from build123d import *

# Parameters (mm, degrees)
SKETCH_1_R          = 1.531489915
EXTRUDE_1_DEPTH     = 1.68
SKETCH_1_R_2        = 1.063949022
EXTRUDE_1_2_DEPTH   = 1.68
SKETCH_1_R_3        = 2.489250022
EXTRUDE_1_3_DEPTH   = 1.68
SKETCH_1_W          = 72.86
SKETCH_1_H          = 61.86
SKETCH_1_R_4        = 1.55
EXTRUDE_1_4_DEPTH   = 1.68
SKETCH_2_R          = 3
SKETCH_2_R_2        = 1.55
EXTRUDE_3_DEPTH     = 2
SKETCH_3_W          = 72.86
SKETCH_3_H          = 61.86
SKETCH_3_W_2        = 69.50125591
SKETCH_3_H_2        = 58.5
EXTRUDE_4_DEPTH     = 15.85
SKETCH_4_W          = 17
SKETCH_4_H          = 15
CUT_EXTRUDE_1_DEPTH = 3.68
SKETCH_6_W          = 7.25
SKETCH_6_H          = 16
SKETCH_6_W_2        = 2.5
SKETCH_6_H_2        = 18
CUT_EXTRUDE_3_DEPTH = 7.8
SKETCH_7_W          = 10
SKETCH_7_H          = 4
SKETCH_7_W_2        = 17
SKETCH_7_H_2        = 8
SKETCH_7_W_3        = 8
SKETCH_7_H_3        = 13.300256909
CUT_EXTRUDE_5_DEPTH = 2
SKETCH_8_R          = 1.556852558
SKETCH_8_W          = 2.041099746
SKETCH_8_H          = 24.945353107
CUT_EXTRUDE_6_DEPTH = 2
FILLET_1_R          = 1.68
FILLET_2_R          = 2
FILLET_3_R          = 1.68
FILLET_4_R          = 2
FILLET_5_R          = 3
FILLET_6_R          = 1
FILLET_7_R          = 1
SKETCH_9_R          = 4
CUT_EXTRUDE_7_DEPTH = 0.8
SKETCH_10_W         = 44.758598589
SKETCH_10_H         = 6.5
SKETCH_10_W_2       = 44.448850503
CUT_EXTRUDE_8_DEPTH = 0.8
SKETCH_11_R         = 1.55
EXTRUDE_6_DEPTH     = 10.65
CUT_EXTRUDE_9_DEPTH = 62.6
FILLET_8_R          = 4
FILLET_9_R          = 1


with BuildPart() as part:
    # 草图1 → 凸台-拉伸1 (new body)
    with BuildSketch(Plane.XY):
        with Locations((1.504266973, 51.672660554)):
            Circle(SKETCH_1_R)
    extrude(amount=EXTRUDE_1_DEPTH)


with BuildPart() as body_2:
    # 草图1 → Extrude 1 2 (new body)
    with BuildSketch(Plane.XY):
        with Locations((-18.258772408, 61.840992468)):
            Circle(SKETCH_1_R_2)
    extrude(amount=EXTRUDE_1_2_DEPTH)


with BuildPart() as body_3:
    # 草图1 → Extrude 1 3 (new body)
    with BuildSketch(Plane.XY):
        with Locations((-18.258772408, -10.975845657)):
            Circle(SKETCH_1_R_3)
    extrude(amount=EXTRUDE_1_3_DEPTH)


with BuildPart() as body_4:
    # 草图1 → Extrude 1 4 (new body)
    with BuildSketch(Plane.XY):
        with Locations((-46.758772408, 26.672660554)):
            Rectangle(SKETCH_1_W, SKETCH_1_H)
        with Locations((-76.258772408, 51.672660554)):
            Circle(SKETCH_1_R_4, mode=Mode.SUBTRACT)
        with Locations((-18.258772408, 51.672660554)):
            Circle(SKETCH_1_R_4, mode=Mode.SUBTRACT)
        with Locations((-76.258772408, 2.672660554)):
            Circle(SKETCH_1_R_4, mode=Mode.SUBTRACT)
        with Locations((-18.258772408, 2.672660554)):
            Circle(SKETCH_1_R_4, mode=Mode.SUBTRACT)
    extrude(amount=EXTRUDE_1_4_DEPTH)

    # 草图2 → 凸台-拉伸3 (add)
    # profile 1 of 4: a face of its own
    with BuildSketch(Plane.XY.offset(1.68)):
        with Locations((-76.258772408, 2.672660554)):
            Circle(SKETCH_2_R)
        with Locations((-76.258772408, 2.672660554)):
            Circle(SKETCH_2_R_2, mode=Mode.SUBTRACT)
    # profile 2 of 4: a face of its own
    with BuildSketch(Plane.XY.offset(1.68)):
        with Locations((-18.258772408, 2.672660554)):
            Circle(SKETCH_2_R)
        with Locations((-18.258772408, 2.672660554)):
            Circle(SKETCH_2_R_2, mode=Mode.SUBTRACT)
    # profile 3 of 4: a face of its own
    with BuildSketch(Plane.XY.offset(1.68)):
        with Locations((-76.258772408, 51.672660554)):
            Circle(SKETCH_2_R)
        with Locations((-76.258772408, 51.672660554)):
            Circle(SKETCH_2_R_2, mode=Mode.SUBTRACT)
    # profile 4 of 4: a face of its own
    with BuildSketch(Plane.XY.offset(1.68)):
        with Locations((-18.258772408, 51.672660554)):
            Circle(SKETCH_2_R)
        with Locations((-18.258772408, 51.672660554)):
            Circle(SKETCH_2_R_2, mode=Mode.SUBTRACT)
    extrude(amount=EXTRUDE_3_DEPTH)

    # 草图3 → 凸台-拉伸4 (add)
    with BuildSketch(Plane.XY.offset(1.68)):
        with Locations((-46.758772408, 26.672660554)):
            Rectangle(SKETCH_3_W, SKETCH_3_H)
        with Locations((-46.758144453, 26.672660554)):
            Rectangle(SKETCH_3_W_2, SKETCH_3_H_2, mode=Mode.SUBTRACT)
    extrude(amount=EXTRUDE_4_DEPTH)

    # 草图4 → 切除-拉伸1 (cut)
    with BuildSketch(Plane(origin=(0, 0, 0), x_dir=(-1, 0, 0), z_dir=(0, 0, -1))):
        with Locations((74.688772408, 28.322197805)):
            Rectangle(SKETCH_4_W, SKETCH_4_H)
    extrude(amount=-CUT_EXTRUDE_1_DEPTH, mode=Mode.SUBTRACT)

    # 草图6 → 切除-拉伸3 (cut)
    with BuildSketch(Plane(origin=(-10.328772408, 0, 0), x_dir=(0, 0, -1), z_dir=(1, 0, 0))):
        with Locations((-8.625, 30.672660554)):
            Rectangle(SKETCH_6_W, SKETCH_6_H)
        with Locations((-14.975303343, 19.628822862)):
            Rectangle(SKETCH_6_W_2, SKETCH_6_H_2)
    extrude(amount=-CUT_EXTRUDE_3_DEPTH, mode=Mode.SUBTRACT)

    # 草图7 → 切除-拉伸5 (cut)
    with BuildSketch(Plane.XZ.offset(4.257339446)):
        with Locations((-69.258772408, 6.68)):
            Rectangle(SKETCH_7_W, SKETCH_7_H)
        with Locations((-47.758772408, 8.68)):
            Rectangle(SKETCH_7_W_2, SKETCH_7_H_2)
        with Locations((-26.258772408, 11.330128455)):
            Rectangle(SKETCH_7_W_3, SKETCH_7_H_3)
    extrude(amount=-CUT_EXTRUDE_5_DEPTH, mode=Mode.SUBTRACT)

    # 草图8 → 切除-拉伸6 (cut)
    with BuildSketch(Plane.ZY.offset(83.188772408)):
        with Locations((7.843859074, 9.687980695)):
            Circle(SKETCH_8_R)
        with Locations((7.730007332, 28.982792683)):
            Rectangle(SKETCH_8_W, SKETCH_8_H)
    extrude(amount=-CUT_EXTRUDE_6_DEPTH, mode=Mode.SUBTRACT)

    # 圆角1
    fillet_1_edges = [body_4.edges().sort_by_distance(p)[0] for p in [
        (-12.007516498, 55.922660554, 9.605),
        (-81.508772408, 55.922660554, 9.605),
        (-81.508772408, -2.577339446, 9.605),
        (-12.007516498, -2.577339446, 9.605),
        (-10.328772408, -4.257339446, 8.765),
        (-83.188772408, -4.257339446, 8.765),
        (-83.188772408, 57.602660554, 8.765),
        (-10.328772408, 57.602660554, 8.765),
    ]]
    fillet(fillet_1_edges, radius=FILLET_1_R)

    # 圆角2
    fillet_2_edges = [body_4.edges().sort_by_distance(p)[0] for p in [
        (-66.188772408, 20.822197805, 0.84),
        (-66.188772408, 35.822197805, 0.84),
    ]]
    fillet(fillet_2_edges, radius=FILLET_2_R)

    # 圆角3
    fillet_3_edges = [body_4.edges().sort_by_distance(p)[0] for p in [
        (-74.258772408, -3.417339446, 4.68),
        (-64.258772408, -3.417339446, 4.68),
    ]]
    fillet(fillet_3_edges, radius=FILLET_3_R)

    # 圆角4
    fillet_4_edges = [body_4.edges().sort_by_distance(p)[0] for p in [
        (-56.258772408, -3.417339446, 4.68),
        (-39.258772408, -3.417339446, 4.68),
    ]]
    fillet(fillet_4_edges, radius=FILLET_4_R)

    # 圆角5
    fillet_5_edges = [body_4.edges().sort_by_distance(p)[0] for p in [
        (-30.258772408, -3.417339446, 4.68),
        (-22.258772408, -3.417339446, 4.68),
    ]]
    fillet(fillet_5_edges, radius=FILLET_5_R)

    # 圆角6
    fillet_6_edges = [body_4.edges().sort_by_distance(p)[0] for p in [
        (-11.168144453, 10.628822862, 16.225303343),
        (-11.168144453, 28.628822862, 16.225303343),
        (-11.168144453, 28.628822862, 13.725303343),
        (-11.168144453, 10.628822862, 13.725303343),
    ]]
    fillet(fillet_6_edges, radius=FILLET_6_R)

    # 圆角7
    fillet_7_edges = [body_4.edges().sort_by_distance(p)[0] for p in [
        (-11.168144453, 38.672660554, 5),
        (-11.168144453, 22.672660554, 5),
        (-11.168144453, 22.672660554, 12.25),
        (-11.168144453, 38.672660554, 12.25),
        (-82.348772408, 16.510116129, 6.709457459),
        (-82.348772408, 41.455469236, 6.709457459),
        (-82.348772408, 41.455469236, 8.750557205),
        (-82.348772408, 16.510116129, 8.750557205),
        (-82.348772408, 20.822197805, 3.68),
        (-82.348772408, 35.822197805, 3.68),
    ]]
    fillet(fillet_7_edges, radius=FILLET_7_R)

    # 草图9 → 切除-拉伸7 (cut)
    with BuildSketch(Plane(origin=(0, 0, 0), x_dir=(-1, 0, 0), z_dir=(0, 0, -1))):
        with Locations((18.258772408, 51.672660554)):
            Circle(SKETCH_9_R)
        with Locations((76.258772408, 51.672660554)):
            Circle(SKETCH_9_R)
        with Locations((18.258772408, 2.672660554)):
            Circle(SKETCH_9_R)
        with Locations((76.258772408, 2.672660554)):
            Circle(SKETCH_9_R)
    extrude(amount=-CUT_EXTRUDE_7_DEPTH, mode=Mode.SUBTRACT)

    # 草图10 → 切除-拉伸8 (cut)
    with BuildSketch(Plane(origin=(0, 0, 0), x_dir=(-1, 0, 0), z_dir=(0, 0, -1))):
        with Locations((41.37196271, 38.672660554)):
            Rectangle(SKETCH_10_W, SKETCH_10_H)
        with Locations((41.37196271, 14.672660554)):
            Rectangle(SKETCH_10_W_2, SKETCH_10_H)
    extrude(amount=-CUT_EXTRUDE_8_DEPTH, mode=Mode.SUBTRACT)

    # 草图11 → 凸台-拉伸6 (add)
    # profile 1 of 2: a face of its own
    with BuildSketch(Plane.XY.offset(3.68)):
        Polygon((-79.828772408, 55.922660554), (-81.508772408, 54.242660554), (-81.508772408, 48.531036753), (-72.875228226, 48.531036753), (-72.875228226, 55.922660554), align=None)
        with Locations(Location((-76.258772408, 51.672660554, 0), (0, 0, 180))):
            Circle(SKETCH_11_R, mode=Mode.SUBTRACT)
    # profile 2 of 2: a face of its own
    with BuildSketch(Plane.XY.offset(3.68)):
        Polygon((-93.925658587, 53.936639744), (-95.605658587, 52.256639744), (-95.605658587, 46.545015943), (-86.972114405, 46.545015943), (-86.972114405, 53.936639744), align=None)
        with Locations(Location((-90.355658587, 49.686639744, 0), (0, 0, 180))):
            Circle(SKETCH_11_R, mode=Mode.SUBTRACT)
    extrude(amount=EXTRUDE_6_DEPTH)


with BuildPart() as extrude_6_piece_1:
    # of the separate pieces the step leaves, piece 1, a body of its own (extrude_6_pieces)
    add(body_4.part.solids().sort_by_distance((-10.328772408, 38.672660554, 6))[0])


with BuildPart() as extrude_6_piece_2:
    # of the separate pieces the step leaves, piece 2, a body of its own (extrude_6_pieces)
    add(body_4.part.solids().sort_by_distance((-93.925658587, 53.936639744, 3.68))[0])

    # 圆角8
    # the kernel refuses this fillet: 4 mm, written as the material it takes off along each edge
    with BuildSketch(Plane(origin=(-93.925658587, 53.936639744, -0.462135624), x_dir=(-0.7071067811865455, -0.7071067811865497, 0), z_dir=(0, 0, 1))) as fillet_8_piece_1:
        with BuildLine():
            CenterArc((FILLET_8_R * 0.414213562373, FILLET_8_R), FILLET_8_R, 225, 45)
            Line((-FILLET_8_R * 0.292893218813, FILLET_8_R * 0.292893218813), (0, 0))
            Line((0, 0), (FILLET_8_R * 0.414213562373, 0))
        make_face()
    extrude(amount=18.934271247, mode=Mode.SUBTRACT)
    with BuildSketch(Plane(origin=(-95.605658587, 52.256639744, -0.462135624), x_dir=(0.7071067811865411, 0.707106781186554, 0), z_dir=(0, 0, 1))) as fillet_8_piece_2:
        with BuildLine():
            CenterArc((FILLET_8_R * 0.414213562373, -FILLET_8_R), FILLET_8_R, 90, 45)
            Line((-FILLET_8_R * 0.292893218813, -FILLET_8_R * 0.292893218813), (0, 0))
            Line((0, 0), (FILLET_8_R * 0.414213562373, 0))
        make_face()
    extrude(amount=18.934271247, mode=Mode.SUBTRACT)

    # 圆角9
    fillet_9_edges = [extrude_6_piece_2.edges().sort_by_distance(p)[0] for p in [
        (-86.972114405, 53.936639744, 9.005),
        (-86.972114405, 46.545015943, 9.005),
        (-95.605658587, 46.545015943, 9.005),
    ]]
    fillet(fillet_9_edges, radius=FILLET_9_R)


with BuildPart() as cut_extrude_9_tool:
    # 草图13 → 切除-拉伸9 (new body)
    with BuildSketch(Plane.XY.offset(17.53)):
        Polygon((-85.534397359, 61.466506159), (-87.240895033, -11.116528255), (-1.802244806, -17.146153371), (14.580132867, 61.466506159), (-40.278079036, 71.546219088), align=None)
    extrude(amount=-CUT_EXTRUDE_9_DEPTH)


with BuildPart() as part_1:
    add(part.part)

    # 切除-拉伸9: cut by cut_extrude_9_tool
    add(cut_extrude_9_tool.part, mode=Mode.SUBTRACT)


with BuildPart() as body_2_1:
    add(body_2.part)

    # 切除-拉伸9: cut by cut_extrude_9_tool
    add(cut_extrude_9_tool.part, mode=Mode.SUBTRACT)


with BuildPart() as body_3_1:
    add(body_3.part)

    # 切除-拉伸9: cut by cut_extrude_9_tool
    add(cut_extrude_9_tool.part, mode=Mode.SUBTRACT)


with BuildPart() as extrude_6_piece_1_1:
    add(extrude_6_piece_1.part)

    # 切除-拉伸9: cut by cut_extrude_9_tool
    add(cut_extrude_9_tool.part, mode=Mode.SUBTRACT)


solid = extrude_6_piece_2.part
Could you check a few things on this model? Use its own coordinates, in mm. Give positions to 0.01 mm unless a question says otherwise; leave off trailing zeros. Order: outer loops, then holes, each group sorted by start corner. A loop starts at its lowest first (then second) coordinate and runs counter-clockwise, first axis right, second up.
1. Thinking about a two-plate mould opening in X: for faces 1 (the cylindrical face through (-91.834, 49.221, 8.93)), 2 (the flat face through (-91, 46.545, 9)), 3 (the cylindrical face through (-87.257, 46.846, 9.08)), which applies, +X half, -X half, draft (parallel to the pull), parting line (faces both ways), or undercut?
Answers below:
face 1: undercut
face 2: draft
face 3: +X half
2. Suppose I cut it at A-A (x = -89.25). Write out the boundary of the cut face in (y, z), plus the area to 3 significant figures.
Answers below:
outline: (46.55, 3.68) - (48.6, 3.68) - (48.6, 14.33) - (46.55, 14.33) - close; (50.77, 3.68) - (53.94, 3.68) - (53.94, 14.33) - (50.77, 14.33) - close
area: 55.6 mm2
3. Suppose I cut it at B-B (y = 49.25). Write out the boundary of the cut face in (x, z).
Answers below:
outline: (-95.61, 3.68) - (-91.84, 3.68) - (-91.84, 14.33) - (-95.61, 14.33) - close; (-88.87, 3.68) - (-86.97, 3.68) - (-86.97, 14.33) - (-88.87, 14.33) - close
4. Suppose I cut it at D-D (y = 52.75). Write out the boundary of the cut face in (x, z).
Answers below:
outline: (-94.98, 3.68) - (-86.97, 3.68) - (-86.97, 14.33) - (-94.98, 14.33) - close
5. For pin 1 (2 mm diameter, centred on x = -94, z = 11.5, fed in from +Y), with a flat end and sliding along its axis, tell me the tip position at first contact or that it passes through.
Answers below:
pin 1: stops at y = 53.87
6. Suppose I cut it at C-C (z = 13.75). Write out the boundary of the cut face in (x, y), plus the area to 3 significant figures.
Answers below:
outline: (-95.61, 47.55) arc R1 ccw to (-94.61, 46.55) - (-87.97, 46.55) arc R1 ccw to (-86.97, 47.55) - (-86.97, 52.94) arc R1 ccw to (-87.97, 53.94) - (-92.27, 53.94) arc R4 ccw to (-94.75, 53.08) arc R4 ccw to (-95.61, 50.6) - close; hole circle Ø3.1 at (-90.36, 49.69)
area: 53.5 mm2
7. I need wall thicknesses on L1, parallel to Y at x = -91, z = 7.5; L2, parallel to X at y = 47.5, z = 9.75; L3, parallel to Y at x = -91.5, z = 14.25. Which ranges of each line are inside material? Lowest first, please.
Answers below:
L1: y = 46.55 to 48.28, 51.1 to 53.94
L2: x = -95.6 to -86.97
L3: y = 46.55 to 48.64, 50.73 to 53.94
